Part model, mm, in its own coordinate system. A direction names the side the tool comes from. Round coordinates to 2 decimals unless told otherwise and drop trailing zeros. Loops run counter-clockwise (first coordinate to the right, second up) from the corner with the lowest first, then second, coordinate; pieces in that order, holes last. Notation, with made-up numbers: (25.25, -21.5) - (33.25, -21.5) arc R13 cw to (33.25, -6.5) - close; hole circle Ø2 at (-33.75, 7). An arc over 180 degrees is marked (long way). Put each result on its own line as item: value.
from build123d import *

# Parameters (mm, degrees)
SKETCH1_W               = 41.275
SKETCH1_H               = 88.9
BOSS_EXTRUDE1_DEPTH     = 5.9944
SKETCH1_5_W             = 8.89
SKETCH1_5_H             = 88.9
BOSS_EXTRUDE2_DEPTH     = 12.3444
SKETCH3_R               = 2.2225
CUT_EXTRUDE1_DEPTH      = 1
CUT_EXTRUDE1_DEPTH_BACK = 13.3444
SKETCH4_R               = 3.683
CUT_EXTRUDE2_DEPTH      = 4.064
SKETCH5_W               = 2.54
SKETCH5_H               = 88.9
CUT_EXTRUDE3_DEPTH      = 7.35
CUT_EXTRUDE3_DEPTH_BACK = 6.9944
SKETCH6_R               = 6.35
CUT_EXTRUDE4_DEPTH      = 1
CUT_EXTRUDE4_DEPTH_BACK = 13.3444


with BuildPart() as part:
    # Sketch1 → Boss-Extrude1 (new body)
    with BuildSketch(Plane(origin=(0, 0, 0), x_dir=(1, 0, 0), z_dir=(0, 1, 0))):
        with Locations((20.6375, 44.45)):
            Rectangle(SKETCH1_W, SKETCH1_H)
    extrude(amount=BOSS_EXTRUDE1_DEPTH)

    # Sketch1<5> → Boss-Extrude2 (add)
    with BuildSketch(Plane(origin=(0, 0, 0), x_dir=(1, 0, 0), z_dir=(0, 1, 0))):
        with Locations((45.72, 44.45)):
            Rectangle(SKETCH1_5_W, SKETCH1_5_H)
    extrude(amount=BOSS_EXTRUDE2_DEPTH)

    # Sketch3 → Cut-Extrude1 (cut, two sides)
    with BuildSketch(Plane(origin=(0, 12.3444, 0), x_dir=(1, 0, 0), z_dir=(0, 1, 0))) as cut_extrude1_sk:
        with Locations((45.72, 82.55)):
            Circle(SKETCH3_R)
        with Locations((45.72, 6.35)):
            Circle(SKETCH3_R)
    extrude(amount=CUT_EXTRUDE1_DEPTH, mode=Mode.SUBTRACT)
    extrude(cut_extrude1_sk.sketch, amount=-CUT_EXTRUDE1_DEPTH_BACK, mode=Mode.SUBTRACT)

    # Sketch4 → Cut-Extrude2 (cut)
    with BuildSketch(Plane.XZ):
        with Locations((45.72, -6.35)):
            Circle(SKETCH4_R)
        with Locations((45.72, -82.55)):
            Circle(SKETCH4_R)
    extrude(amount=-CUT_EXTRUDE2_DEPTH, mode=Mode.SUBTRACT)

    # Sketch5 → Cut-Extrude3 (cut, two sides)
    with BuildSketch(Plane(origin=(0, 5.9944, 0), x_dir=(1, 0, 0), z_dir=(0, 1, 0))) as cut_extrude3_sk:
        with Locations((1.27, 44.45)):
            Rectangle(SKETCH5_W, SKETCH5_H)
    extrude(amount=CUT_EXTRUDE3_DEPTH, mode=Mode.SUBTRACT)
    extrude(cut_extrude3_sk.sketch, amount=-CUT_EXTRUDE3_DEPTH_BACK, mode=Mode.SUBTRACT)

    # Sketch6 → Cut-Extrude4 (cut, two sides)
    with BuildSketch(Plane(origin=(0, 12.3444, 0), x_dir=(1, 0, 0), z_dir=(0, 1, 0))) as cut_extrude4_sk:
        with Locations((50.165, 43.18)):
            Circle(SKETCH6_R)
    extrude(amount=CUT_EXTRUDE4_DEPTH, mode=Mode.SUBTRACT)
    extrude(cut_extrude4_sk.sketch, amount=-CUT_EXTRUDE4_DEPTH_BACK, mode=Mode.SUBTRACT)


solid = part.part
1. Band-saw the part on C-C (x = 47). List the corners of the cut face in (y, z), plus the area to 3 significant figures.
A:
outline: (0, -88.9) - (12.34, -88.9) - (12.34, -84.37) - (4.06, -84.37) - (4.06, -86) - (0, -86) - close; (0, -79.1) - (4.06, -79.1) - (4.06, -80.73) - (12.34, -80.73) - (12.34, -48.69) - (0, -48.69) - close; (0, -37.67) - (12.34, -37.67) - (12.34, -8.17) - (4.06, -8.17) - (4.06, -9.8) - (0, -9.8) - close; (0, -2.9) - (4.06, -2.9) - (4.06, -4.53) - (12.34, -4.53) - (12.34, 0) - (0, 0) - close
area: 845 mm²
2. Two-plate mould, pull along X, no slides. Class faces 1 (the flat face through (22, 5.994, -45)), 2 (the cylindrical face through (43.5, 8.3, -6.4)), 3 (the flat face through (50.165, 6, -69)): pulls with the +X half, pulls with the -X half, needs draft (parallel to the pull), parting line crosses it, or undercut.
A:
face 1: needs draft
face 2: undercut
face 3: pulls with the +X half
3. Tool access for faces 4 (the flat face through (31, 3, 0)), 5 (the cylindrical face through (47.419, 2.004, -85.817)), 6 (the flat face through (41.275, 9, -44)): list every direction of +Z, -Z, +X, -X, +Y, -Y with a clear straight run to the whole face (end or side of a thin tool).
A:
face 4: +Z, +X, -X, +Y, -Y
face 5: -Y
face 6: +Z, -Z, -X, +Y
4. Band-saw the part on B-B (y = 9). Give the number of separate pieces and of enclosed holes in the cut face, plus the area to 3 significant figures.
A:
separate pieces: 1
enclosed holes: 2
area: 696 mm²
5. Band-saw the part on A-A (z = -82.55). List the corners of the cut face in (x, y) (1 decimal).
A:
outline: (2.5, 0) - (42, 0) - (42, 4.1) - (43.5, 4.1) - (43.5, 12.3) - (41.3, 12.3) - (41.3, 6) - (2.5, 6) - close; (47.9, 4.1) - (49.4, 4.1) - (49.4, 0) - (50.2, 0) - (50.2, 12.3) - (47.9, 12.3) - close
6. Pin check, flat tips, straight feed: P1, Ø6, axis at x = 45.72, z = -82.55, coming from the -Y side; P2, Ø1.9, axis at y = 9.5, z = -43, coming from the -X side (3 decimals); P3, Ø2, axis at x = 24, z = -10, coming from the +Y side. Stop position of each tip, or through.
A:
P1: stops at y = 4.06
P2: stops at x = 41.275
P3: stops at y = 5.99
7. Probe line 1 along X through (y, z) = (8.25, -6.35) (1 decimal); line 2 along Z through (x, y) = (45.72, 2.35); line 3 along Y through (x, z) = (17, -61). List the from-to ranges inside material, lowest first. Write a range as [from, to].
A:
line 1: x = [41.3, 43.5], [47.9, 50.2]
line 2: z = [-88.9, -86.23], [-78.87, -47.71], [-38.65, -10.03], [-2.67, 0]
line 3: y = [0, 5.99]
8. Band-saw the part on D-D (z = -15). List the corners of the cut face in (x, y) (3 decimals).
A:
outline: (2.54, 0) - (50.165, 0) - (50.165, 12.344) - (41.275, 12.344) - (41.275, 5.994) - (2.54, 5.994) - close
